from build123d import *

# Parameters (mm, degrees)
SKETCH_1_R      = 2.75
SKETCH_1_R_2    = 4
SKETCH_1_R_3    = 1.283558174
EXTRUDE_1_DEPTH = 3


with BuildPart() as part:
    # 草图1 → 凸台-拉伸1 (new body)
    with BuildSketch(Plane(origin=(0, 0, 0), x_dir=(1, 0, 0), z_dir=(0, 1, 0))):
        with BuildLine():
            ThreePointArc((-65, 20), (-63.535533906, 23.535533906), (-60, 25))
            Line((-60, 25), (0, 25))
            Line((0, 25), (60, 25))
            ThreePointArc((60, 25), (63.535533906, 23.535533906), (65, 20))
            Line((65, 20), (65, -20))
            ThreePointArc((65, -20), (63.535533906, -23.535533906), (60, -25))
            Line((60, -25), (-60, -25))
            ThreePointArc((-60, -25), (-63.535533906, -23.535533906), (-65, -20))
            Line((-65, -20), (-65, 20))
        make_face()
        with Locations(Location((-50, 16, 0), (0, 0, 270))):
            Circle(SKETCH_1_R, mode=Mode.SUBTRACT)
        with Locations(Location((0, 0, 0), (0, 0, 270))):
            Circle(SKETCH_1_R_2, mode=Mode.SUBTRACT)
        with Locations(Location((15.5, 15.5, 0), (0, 0, 270))):
            Circle(SKETCH_1_R_3, mode=Mode.SUBTRACT)
        with Locations(Location((15.5, -15.5, 0), (0, 0, 270))):
            Circle(SKETCH_1_R_3, mode=Mode.SUBTRACT)
        with Locations(Location((-15.5, -15.5, 0), (0, 0, 270))):
            Circle(SKETCH_1_R_3, mode=Mode.SUBTRACT)
        with Locations(Location((-15.5, 15.5, 0), (0, 0, 270))):
            Circle(SKETCH_1_R_3, mode=Mode.SUBTRACT)
        with Locations(Location((50, 0, 0), (0, 0, 270))):
            Circle(SKETCH_1_R_2, mode=Mode.SUBTRACT)
        with Locations(Location((50, 16, 0), (0, 0, 270))):
            Circle(SKETCH_1_R, mode=Mode.SUBTRACT)
        with Locations(Location((50, -16, 0), (0, 0, 270))):
            Circle(SKETCH_1_R, mode=Mode.SUBTRACT)
        with Locations(Location((-50, -16, 0), (0, 0, 270))):
            Circle(SKETCH_1_R, mode=Mode.SUBTRACT)
        with Locations(Location((-50, 0, 0), (0, 0, 270))):
            Circle(SKETCH_1_R_2, mode=Mode.SUBTRACT)
    extrude(amount=EXTRUDE_1_DEPTH)


solid = part.part
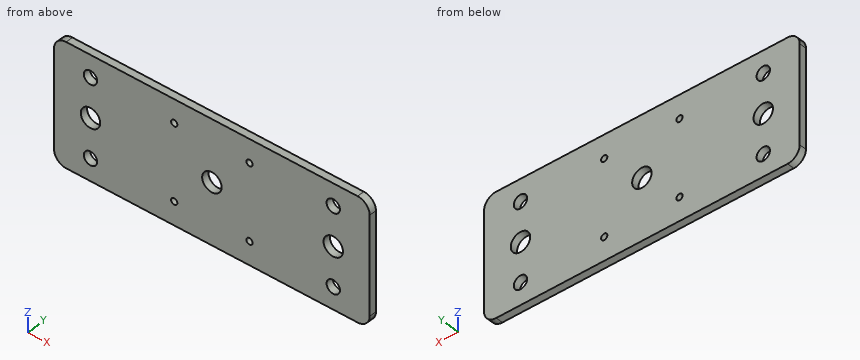
Work out the finished part from the listing and answer in its coordinate system (mm). Round coordinates to 2 decimals unless told otherwise and drop trailing zeros. Write each loop counter-clockwise with the first axis right and the second up, starting at its lowest first coordinate (ties: lowest second). Pieces come first, ordered by that corner, then holes.
1) A cutting plane is placed at D-D (x = 0). Give the vertices of the cut face in (y, z).
2) A cutting plane is placed at A-A (x = -15.5). Give the vertices of the cut face in (y, z), plus the area to 3 significant figures.
3) Straight lines are drawn through the part: line 1 (X direction, y = 1.3, z = -16.5); line 2 (Z direction, x = 16.5, y = 1.9); line 3 (X direction, y = 1, z = -2). For each, find the intervals that lie inside material, in ascending order.
4) A cutting plane is placed at B-B (y = 2.15). Give the number of separate pieces and of enclosed holes in the cut face, plus the area to 3 significant figures.
5) A cutting plane is placed at C-C (z = 2). Give the vertices of the cut face in (x, y).
Completed:
1. outline: (0, -25) - (3, -25) - (3, -4) - (0, -4) - close; (0, 4) - (3, 4) - (3, 25) - (0, 25) - close
2. outline: (0, -25) - (3, -25) - (3, -16.78) - (0, -16.78) - close; (0, -14.22) - (3, -14.22) - (3, 14.22) - (0, 14.22) - close; (0, 16.78) - (3, 16.78) - (3, 25) - (0, 25) - close
2. area: 135 mm2
3. line 1: x = -65 to -52.7, -47.3 to -16.3, -14.7 to 14.7, 16.3 to 47.3, 52.7 to 65
3. line 2: z = -25 to -16.3, -14.7 to 14.7, 16.3 to 25
3. line 3: x = -65 to -53.46, -46.54 to -3.46, 3.46 to 46.54, 53.46 to 65
4. separate pieces: 1
4. enclosed holes: 11
4. area: 6,210 mm2
5. outline: (-65, 0) - (-53.46, 0) - (-53.46, 3) - (-65, 3) - close; (-46.54, 0) - (-3.46, 0) - (-3.46, 3) - (-46.54, 3) - close; (3.46, 0) - (46.54, 0) - (46.54, 3) - (3.46, 3) - close; (53.46, 0) - (65, 0) - (65, 3) - (53.46, 3) - close
